Check sheet for the modelled part. Datum: model origin and axes. Units: mm. A direction names the side the tool comes from. Give positions to 0.01 mm unless a question says otherwise; leave off trailing zeros. Loops run counter-clockwise (first coordinate to the right, second up) from the corner with the lowest first, then second, coordinate; pieces in that order, holes last.
```python
from build123d import *

# Parameters (mm, degrees)
BOSS_EXTRUDE1_DEPTH      = 20.2
BOSS_EXTRUDE1_DEPTH_BACK = 15
SKETCH1_W                = 93.989323661
SKETCH1_H                = 75.639027137
SKETCH1_R                = 28.60558576
CUT_EXTRUDE1_DEPTH       = 65.815428125
CUT_EXTRUDE1_DEPTH_BACK  = 65.815428125
SKETCH7_W                = 73.626868744
SKETCH7_H                = 46
CUT_EXTRUDE2_DEPTH       = 71.936871393
CUT_EXTRUDE2_DEPTH_BACK  = 71.936871393
SKETCH8_W                = 2.074297069
SKETCH8_H                = 75.639027137
CUT_EXTRUDE3_DEPTH       = 92.182778922
CUT_EXTRUDE3_DEPTH_BACK  = 92.182778922
SKETCH9_R                = 9.85217033
SKETCH9_R_2              = 8.836553466


with BuildPart() as part:
    # Sketch1 → Boss-Extrude1 (new, two sides: drawn at the far end of the back side and taken through both)
    # profile 1 of 2: a face of its own
    with BuildSketch(Plane(origin=(0, 0, 0), x_dir=(1, 0, 0), z_dir=(0, 1, 0)).offset(-BOSS_EXTRUDE1_DEPTH_BACK)):
        with Locations((-0.250713069, 1.688387839)):
            Rectangle(SKETCH1_W, SKETCH1_H)
        Polygon((-15.47568065, 38.452030524), (-15.44512512, 38.452030524), (17.164906021, 38.452030524), (43.185007565, 38.452030524), (45.754987202, 38.452030524), (45.754987202, 32.455155104), (45.754987202, 32.45391936), (45.754987202, -35.17483185), (17.616871532, -35.17483185), (-15.375759604, -35.17483185), (-46.245033324, -35.17483185), (-46.245033324, 38.452030524), (-43.675074212, 38.452030524), align=None, mode=Mode.SUBTRACT)
    # profile 2 of 2: a face of its own
    with BuildSketch(Plane(origin=(0, 0, 0), x_dir=(1, 0, 0), z_dir=(0, 1, 0)).offset(-BOSS_EXTRUDE1_DEPTH_BACK)):
        Polygon((17.164906021, 38.452030524), (-15.44512512, 38.452030524), (-15.47568065, 38.452030524), (-43.675074212, 38.452030524), (-46.245033324, 38.452030524), (-46.245033324, -35.17483185), (-15.375759604, -35.17483185), (17.616871532, -35.17483185), (45.754987202, -35.17483185), (45.754987202, 32.45391936), (45.754987202, 32.455155104), (45.754987202, 38.452030524), (43.185007565, 38.452030524), align=None)
        with Locations(Location((-0.126795962, 0.062260433, 0), (0, 0, 270))):
            Circle(SKETCH1_R, mode=Mode.SUBTRACT)
    extrude(amount=BOSS_EXTRUDE1_DEPTH + BOSS_EXTRUDE1_DEPTH_BACK)

    # Sketch7 → Cut-Extrude1 (cut, two sides: drawn at the far end of the back side and taken through both)
    with BuildSketch(Plane(origin=(0, 0, 0), x_dir=(0, 0, -1), z_dir=(1, 0, 0)).offset(-CUT_EXTRUDE1_DEPTH_BACK)):
        with Locations((1.63860241, -3.238314763)):
            Rectangle(SKETCH7_W, SKETCH7_H)
    extrude(amount=CUT_EXTRUDE1_DEPTH + CUT_EXTRUDE1_DEPTH_BACK, mode=Mode.SUBTRACT)

    # Sketch8 → Cut-Extrude2 (cut, two sides: drawn at the far end of the back side and taken through both)
    with BuildSketch(Plane(origin=(0, 20.2, 0), x_dir=(1, 0, 0), z_dir=(0, 1, 0)).offset(-CUT_EXTRUDE2_DEPTH_BACK)):
        with Locations((-46.208226366, 1.688387839)):
            Rectangle(SKETCH8_W, SKETCH8_H)
    extrude(amount=CUT_EXTRUDE2_DEPTH + CUT_EXTRUDE2_DEPTH_BACK, mode=Mode.SUBTRACT)

    # Sketch9 → Cut-Extrude3 (cut, two sides: drawn at the far end of the back side and taken through both)
    with BuildSketch(Plane.XY.offset(36.131125729).offset(-CUT_EXTRUDE3_DEPTH_BACK)):
        with Locations((30.686426908, 3.531311209)):
            Circle(SKETCH9_R)
        with Locations((-24.996180107, 3.923442244)):
            Circle(SKETCH9_R_2)
    extrude(amount=CUT_EXTRUDE3_DEPTH + CUT_EXTRUDE3_DEPTH_BACK, mode=Mode.SUBTRACT)


solid = part.part
```
(1) Material ranges on line 1 (Z direction, x = 19, y = 3.5); line 2 (Y direction, x = 23.5, z = 28.5), recorded low to high.
(2) Gauge pin test, flat ends, axial feed: pin 1 Ø12 at (y, z) = (14, 6.5) entering from -X; pin 2 Ø8 at (y, z) = (12.5, 5) entering from +X. Record the tip position at first contact, or that the pin passes through.
(3) Section check D-D on x = 30.5. Record the boundary of the cut face in (y, z), plus the area to 3 significant figures.
(4) Section check C-C on z = -23.5. Record the boundary of the cut face in (x, y).
(5) Section check A-A on y = -11.5. Record the boundary of the cut face in (x, z), plus the area to 3 significant figures.
(6) Release check for a two-part mould opening along Z. For faces 1 (the face through (0, 2, -38.452)), 2 (the face through (20.844, 3.964, 35.646)), 3 (the face through (0, 2, 36.131)) record: pulls with the +Z half, pulls with the -Z half, needs draft (parallel to the pull), parting line crosses it, or undercut.
(7) Access from +Z, -Z, +X, -X, +Y, -Y to the whole of each face (thin tool, end or side, straight path). Record for faces 4 (the face through (0, 2, 35.175)), 5 (the face through (0, 2, -39.508)).
(8) Section check B-B on x = -2.5. Record the boundary of the cut face in (y, z), plus the area to 3 significant figures.
Computed values:
1. line 1: z = -39.51 to -38.45, 35.17 to 36.13
1. line 2: y = 19.76 to 20.2
2. pin 1: stops at x = -45.17
2. pin 2: passes through
3. outline: (-15, -39.51) - (-6.32, -39.51) - (-6.32, -38.45) - (-15, -38.45) - close; (-15, 35.17) - (-6.32, 35.17) - (-6.32, 36.13) - (-15, 36.13) - close; (13.38, -39.51) - (20.2, -39.51) - (20.2, 36.13) - (13.38, 36.13) - (13.38, 35.17) - (19.76, 35.17) - (19.76, -38.45) - (13.38, -38.45) - close
3. area: 63.5 mm2
4. outline: (-45.17, 19.76) - (-16.53, 19.76) - (-16.53, 20.2) - (-45.17, 20.2) - close; (16.27, 19.76) - (46.74, 19.76) - (46.74, 20.2) - (16.27, 20.2) - close
5. outline: (-45.17, -39.51) - (46.74, -39.51) - (46.74, -38.45) - (-45.17, -38.45) - close; (-45.17, 35.17) - (46.74, 35.17) - (46.74, 36.13) - (-45.17, 36.13) - close
5. area: 185 mm2
6. face 1: undercut
6. face 2: needs draft
6. face 3: pulls with the +Z half
7. face 4: +X, -X, -Y
7. face 5: -Z, +X, -X, +Y, -Y
8. outline: (-15, -39.51) - (20.2, -39.51) - (20.2, -28.57) - (19.76, -28.57) - (19.76, -38.45) - (-15, -38.45) - close; (-15, 35.17) - (19.76, 35.17) - (19.76, 28.44) - (20.2, 28.44) - (20.2, 36.13) - (-15, 36.13) - close
8. area: 78.1 mm2
